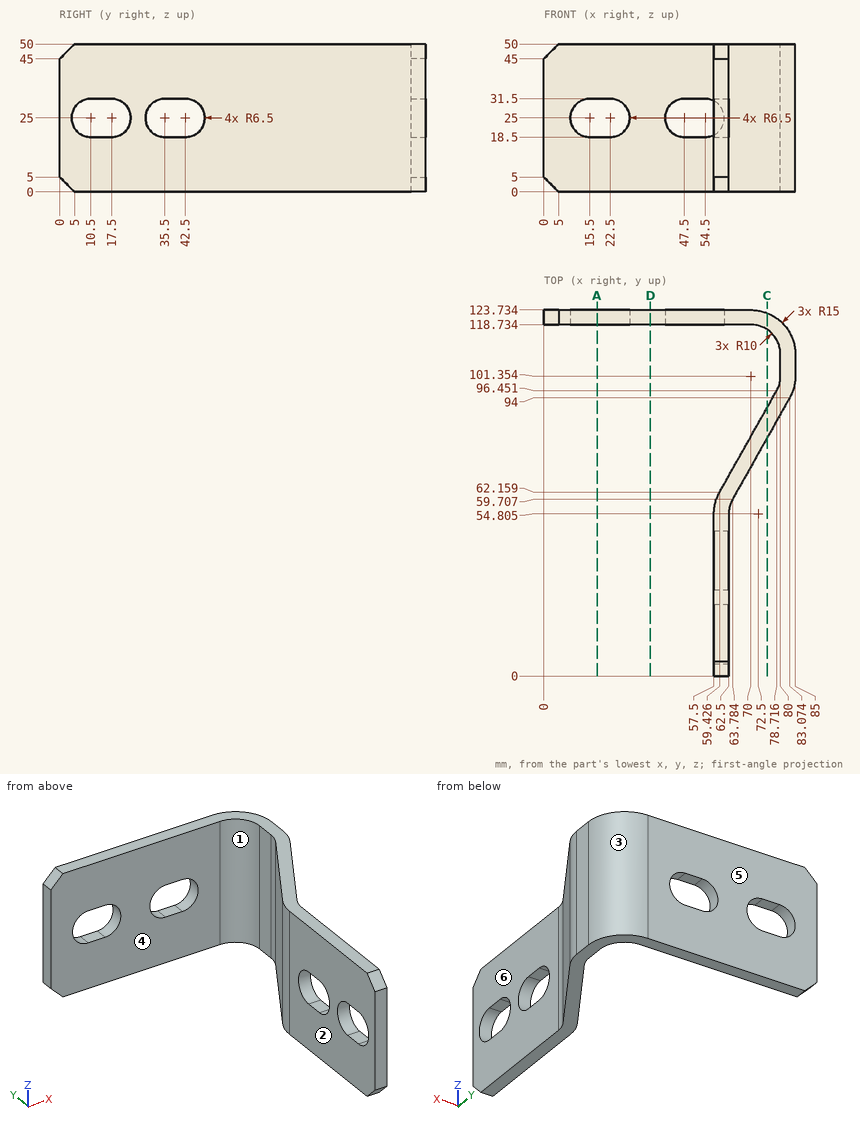
Geometry check sheet. Reference: drawing and pictorial views, mm from the part's lowest x, y, z. A direction names the side the tool comes from. Round coordinates to 2 decimals unless told otherwise and drop trailing zeros. Order: outer loops, then holes, each group sorted by start corner. A loop starts at its lowest first (then second) coordinate and runs counter-clockwise, first axis right, second up. Notation, with made-up numbers: (35, 83) -> (52, 83) arc R24 ccw to (52, 120) -> close; hole circle Ø7 at (41.5, -14.5). An arc over 180 degrees is marked (long way). One line per item, written item: value. Start each with the question number.
Q1. Cross-section at D-D (x = 36). Record the boundary of the cut face in (y, z).
Q2. Thickness scan on line 1 (Y direction, x = 12, z = 38); line 2 (X direction, y = 16, z = 9.5); line 3 (Y direction, x = 67, z = 16) (1 decimal). Record the ranges inside material, lowest first.
Q3. Cross-section at A-A (x = 18). Record the boundary of the cut face in (y, z), and give its area (3 significant figures).
Q4. Set-up check for the marked faces 4, 5 and 6: record each of +Z, -Z, +X, -X, +Y, -Y from which the full face is reachable in a straight line by a thin tool's end or side.
Q5. Gauge pin test, flat ends, axial feed: pin 1 Ø15 at (x, z) = (26, 33) entering from -Y; pin 2 Ø8 at (y, z) = (77, 42) entering from +X; pin 3 Ø25 at (y, z) = (33.5, 19) entering from -X. Record the tip position at first contact, or that the pin passes through.
Q6. Mould release check, pull along Y, two halves, no side actions. Record for the marked faces 1, 2 and 3: pulls with the +Y half, pulls with the -Y half, needs draft (parallel to the pull), parting line crosses it, or undercut.
Q7. Cross-section at C-C (x = 75.5). Record the boundary of the cut face in (y, z) (1 decimal).
Completed:
1. outline: (118.73, 0) -> (123.73, 0) -> (123.73, 50) -> (118.73, 50) -> close
2. line 1: y = 118.73 to 123.73
2. line 2: x = 57.5 to 62.5
2. line 3: y = 65.4 to 75.6, 118.7 to 123.7
3. outline: (118.73, 0) -> (123.73, 0) -> (123.73, 18.5) -> (118.73, 18.5) -> close; (118.73, 31.5) -> (123.73, 31.5) -> (123.73, 50) -> (118.73, 50) -> close
3. area: 185 mm²
4. face 4: +Z, -Z, -X
4. face 5: +Z, -Z, +X, -X, +Y
4. face 6: +Z, -Z, +X, -Y
5. pin 1: stops at y = 118.73
5. pin 2: stops at x = 75.76
5. pin 3: stops at x = 57.5
6. face 1: undercut
6. face 2: needs draft
6. face 3: pulls with the +Y half
7. outline: (80.5, 0) -> (90.7, 0) -> (90.7, 50) -> (80.5, 50) -> close; (117.1, 0) -> (122.7, 0) -> (122.7, 50) -> (117.1, 50) -> close
